Geometry: final body of the model. Coordinates: model frame, mm. Face numbers are marked on the shaded views. Round coordinates to 2 decimals unless told otherwise and drop trailing zeros. Loops run counter-clockwise (first coordinate to the right, second up) from the corner with the lowest first, then second, coordinate; pieces in that order, holes last. Notation, with made-up numbers: (-9, -28.5) - (11, -28.5) arc R34 ccw to (11, 10.5) - close; hole circle Ø9 at (-7.75, 26.25). An arc over 180 degrees is marked (long way). Return JSON: item names as keys, results as strings. Group by question number.
1. Section C-C on z = 3.6. Return loops of the section in (x, y).
2. Section B-B on y = 2.25. Return loops of the section in (x, z).
3. First-contact query: pin 1 Ø1 at (x, z) = (0, 3) entering from -Y; pin 2 Ø1 at (y, z) = (6.5, 1.5) entering from -X; pin 3 Ø1.5 at (x, z) = (-7, 1) entering from +Y. Flat tips, straight axial feed; report the tip coordinate or a pass-through.
4. Draft query along X for the marked faces 1, 2 and 3. Return one class per face: +X half, -X half, draft (parallel to the pull), parting line (faces both ways), or undercut.
5. Section D-D on y = 5.75. Count the separate pieces of the cut face and the enclosed holes in it, and give its area (3 significant figures).
6. Section A-A on x = 0. Return loops of the section in (y, z), and give its area (3 significant figures).
7. Material intervals for probe 1 along Z at (x, y) = (0, 15.55); probe 2 along X at (y, z) = (3, 2.85); probe 3 along X at (y, z) = (12.5, 1.1), sorted ascending.
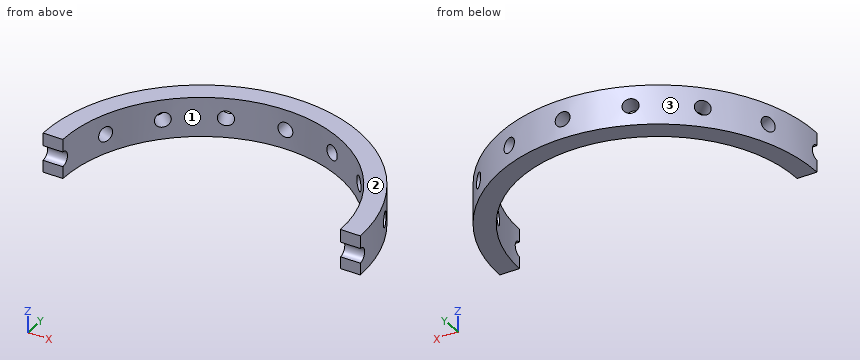
from build123d import *

# Parameters (mm, degrees)
SKETCH_1_R               = 16
SKETCH_1_R_2             = 14
EXTRUDE_1_DEPTH          = 4
SKETCH_2_R               = 0.75
CUT_EXTRUDE_1_DEPTH      = 17
PATTERN_CIRCULAR_1_COUNT = 16
SKETCH_3_W               = 36.79853237
SKETCH_3_H               = 11.94610836
CUT_EXTRUDE_2_DEPTH      = 17.0000001


with BuildPart() as part:
    # ｽｹｯﾁ1 → ﾎﾞｽ - 押し出し1 (new body)
    with BuildSketch(Plane.XY):
        Circle(SKETCH_1_R)
        Circle(SKETCH_1_R_2, mode=Mode.SUBTRACT)
    extrude(amount=EXTRUDE_1_DEPTH)

    # ｽｹｯﾁ2 → ｶｯﾄ - 押し出し1 (cut, through all)
    with BuildSketch(Plane(origin=(0, 0, 0), x_dir=(1, 0, 0), z_dir=(0, 1, 0))):
        with Locations((0, -1.957637914)):
            Circle(SKETCH_2_R)
    cut_extrude_1 = extrude(amount=-CUT_EXTRUDE_1_DEPTH, mode=Mode.SUBTRACT)

    # 円形ﾊﾟﾀｰﾝ1: ｶｯﾄ - 押し出し1 ×16 about axis
    pattern_circular_1_axis = Axis((0, 0, 0), (0, 0, 1))
    for i in range(1, PATTERN_CIRCULAR_1_COUNT):
        add(cut_extrude_1.rotate(pattern_circular_1_axis, i * 360 / PATTERN_CIRCULAR_1_COUNT), mode=Mode.SUBTRACT)

    # ｽｹｯﾁ3 → ｶｯﾄ - 押し出し2 (cut, through all)
    with BuildSketch(Plane(origin=(0, 0, 0), x_dir=(1, 0, 0), z_dir=(0, 1, 0))):
        with Locations((0, -2.028241391)):
            Rectangle(SKETCH_3_W, SKETCH_3_H)
    extrude(amount=-CUT_EXTRUDE_2_DEPTH, mode=Mode.SUBTRACT)


solid = part.part
Taken from the geometry:
{
 "1": {"outline": "(-16, 0) - (-14, 0) arc R14 cw to (14, 0) - (16, 0) arc R16 ccw to start"},
 "2": {"outline": "(-15.84, 0) - (-13.82, 0) - (-13.82, 4) - (-15.84, 4) - close; (13.82, 0) - (15.84, 0) - (15.84, 4) - (13.82, 4) - close"},
 "3": {"pin 1": "y = 13.99", "pin 2": "x = -14.79", "pin 3": "y = 14.73"},
 "4": {"face 1": "undercut", "face 2": "draft", "face 3": "parting line"},
 "5": {"separate pieces": "4", "enclosed holes": "0", "area": "11.2 mm2"},
 "6": {"outline": "(14, 0) - (16, 0) - (16, 1.21) - (14, 1.21) - close; (14, 2.71) - (16, 2.71) - (16, 4) - (14, 4) - close", "area": "5.00 mm2"},
 "7": {"probe 1": "0 to 1.21, 2.71 to 4", "probe 2": "-15.72 to -13.67, 13.67 to 15.72", "probe 3": "-9.99 to -6.3, 6.3 to 9.99"}
}
